Design review of the part built by this model. Coordinates are the model's own, in mm. A direction names the side the tool comes from. Give positions to 0.01 mm unless a question says otherwise; leave off trailing zeros. Loops run counter-clockwise (first coordinate to the right, second up) from the corner with the lowest first, then second, coordinate; pieces in that order, holes last. Notation, with made-up numbers: (-34, 13.25) -> (12, 13.25) arc R21 ccw to (12, 36.25) -> close; hole circle Ø8 at (8, 9). An arc over 180 degrees is marked (long way). Answer as CSV lines item,"result".
from build123d import *

# Parameters (mm, degrees)
BOSS_EXTRUDE1_DEPTH     = 30
CUT_EXTRUDE1_DEPTH      = 74.654599313
CUT_EXTRUDE1_DEPTH_BACK = 74.654599313
SKETCH3_W               = 18
SKETCH3_H               = 30
SKETCH4_R               = 20
SKETCH4_R_2             = 8
BOSS_EXTRUDE2_DEPTH     = 22
CUT_EXTRUDE2_DEPTH      = 12
CUT_EXTRUDE3_DEPTH      = 94.214805691
CUT_EXTRUDE3_DEPTH_BACK = 94.214805691
SKETCH6_R               = 8


with BuildPart() as part:
    # Sketch1 → Boss-Extrude1 (new, symmetric)
    with BuildSketch(Plane.XY):
        Polygon((-45, 0), (45, 0), (25, 50), (-25, 50), align=None)
    extrude(amount=BOSS_EXTRUDE1_DEPTH, both=True)

    # Sketch3 → Cut-Extrude1 (cut, two sides: drawn at the far end of the back side and taken through both)
    with BuildSketch(Plane(origin=(0, 0, 0), x_dir=(0, 0, -1), z_dir=(1, 0, 0)).offset(-CUT_EXTRUDE1_DEPTH_BACK)):
        with Locations((21, 35)):
            Rectangle(SKETCH3_W, SKETCH3_H)
        with Locations((-21, 35)):
            Rectangle(SKETCH3_W, SKETCH3_H)
    extrude(amount=CUT_EXTRUDE1_DEPTH + CUT_EXTRUDE1_DEPTH_BACK, mode=Mode.SUBTRACT)

    # Sketch4 → Boss-Extrude2 (add, symmetric)
    with BuildSketch(Plane.XY):
        with Locations((0, 50)):
            Circle(SKETCH4_R)
        with Locations((0, 50)):
            Circle(SKETCH4_R_2, mode=Mode.SUBTRACT)
    extrude(amount=BOSS_EXTRUDE2_DEPTH, both=True)

    # Sketch5 → Cut-Extrude2 (cut, symmetric)
    with BuildSketch(Plane.XY):
        with BuildLine():
            Line((-20, 50), (-10, 50))
            Line((-10, 50), (-10, 67.320508076))
            ThreePointArc((-10, 67.320508076), (-17.320508076, 60), (-20, 50))
        make_face()
        with BuildLine():
            Line((10, 50), (10, 67.320508076))
            ThreePointArc((10, 67.320508076), (17.320508076, 60), (20, 50))
            Line((20, 50), (10, 50))
        make_face()
    extrude(amount=CUT_EXTRUDE2_DEPTH, both=True, mode=Mode.SUBTRACT)

    # Sketch6 → Cut-Extrude3 (cut, two sides: drawn at the far end of the back side and taken through both)
    with BuildSketch(Plane.XY.offset(12).offset(-CUT_EXTRUDE3_DEPTH_BACK)):
        with Locations((0, 50)):
            Circle(SKETCH6_R)
    extrude(amount=CUT_EXTRUDE3_DEPTH + CUT_EXTRUDE3_DEPTH_BACK, mode=Mode.SUBTRACT)


solid = part.part
Q1. We need section A-A, the plane z = -16.5. State the section outline as (x, y) points.
Filled sheet:
outline,"(-45, 0) -> (45, 0) -> (37, 20) -> (-37, 20) -> close; circle Ø40 at (0, 50); hole circle Ø16 at (0, 50)"
Q2. For faces 5 (the flat face through (-1, 28, 12)), 6 (the cylindrical face through (-2.6, 69.83, 0.31)), 7 (the flat face through (14, 57, 12)), 8 (the flat face through (-14, 57, -12)), list the 3-axis set-ups (+Z, -Z, +X, -X, +Y, -Y) from which the entire face can be reached by the end or side of a thin tool; tool diameter is ignored.
Filled sheet:
face 5,"+Z"
face 6,"none"
face 7,"+X, +Y"
face 8,"-X, +Y"
Q3. Clearance check with flat-ended pins moving along their axes: pin 1 Ø8 at (y, z) = (58.5, -20.5) entering from +X; pin 2 Ø10 at (y, z) = (38.5, 3) entering from -X; pin 3 Ø10 at (y, z) = (54, -21) entering from -X. State where each tip first meets the part, or that it passes through.
Filled sheet:
pin 1,"stops at x = 19.49"
pin 2,"stops at x = -31.6"
pin 3,"stops at x = -20"
Q4. We need section B-B, the plane x = 0. State the section outline as (y, z) points.
Filled sheet:
outline,"(0, -30) -> (20, -30) -> (20, -12) -> (30, -12) -> (30, -22) -> (42, -22) -> (42, 22) -> (30, 22) -> (30, 12) -> (20, 12) -> (20, 30) -> (0, 30) -> close; (58, -22) -> (70, -22) -> (70, 22) -> (58, 22) -> close"
Q5. We need section D-D, the plane y = 39.5. State the section outline as (x, z) points.
Filled sheet:
outline,"(-29.2, -12) -> (-17.02, -12) -> (-17.02, -22) -> (17.02, -22) -> (17.02, -12) -> (29.2, -12) -> (29.2, 12) -> (17.02, 12) -> (17.02, 22) -> (-17.02, 22) -> (-17.02, 12) -> (-29.2, 12) -> close"
Q6. The part is to be moulded in two halves that separate along Y. For faces 1 (the flat face through (18, 50, 0)), 2 (the flat face through (-1, 20, 21)), 3 (the flat face through (-1, 0, 0)), 4 (the flat face through (14, 57, -12)), say which applies: pulls with the +Y half, pulls with the -Y half, needs draft (parallel to the pull), parting line crosses it, or undercut.
Filled sheet:
face 1,"pulls with the +Y half"
face 2,"undercut"
face 3,"pulls with the -Y half"
face 4,"needs draft"
Q7. We need section C-C, the plane x = 21.5. State the section outline as (y, z) points.
Filled sheet:
outline,"(0, -30) -> (20, -30) -> (20, -12) -> (50, -12) -> (50, 12) -> (20, 12) -> (20, 30) -> (0, 30) -> close"
Q8. To check wall thickness, follow probe 1 along Y at (x, z) = (0, -11); probe 2 along X at (y, z) = (50.5, 9); probe 3 along Y at (x, z) = (26, -19). State the ranges of each line that lie inside material, in increasing order. Write a range as from..to.
Filled sheet:
probe 1,"y = 0..42, 58..70"
probe 2,"x = -10..-7.98, 7.98..10"
probe 3,"y = 0..20"
